Check sheet for the modelled part. Datum: model origin and axes. Units: mm. Face numbers are marked on the shaded views. A direction names the side the tool comes from. Give positions to 0.01 mm unless a question says otherwise; leave off trailing zeros. Order: outer loops, then holes, each group sorted by start corner. A loop starts at its lowest first (then second) coordinate and runs counter-clockwise, first axis right, second up.
Item 1: Gauge pin test, flat ends, axial feed: P1, Ø2, axis at y = 22.5, z = -3, coming from the +X side; P2, Ø3, axis at x = -14, z = -1, coming from the -Y side; P3, Ø1, axis at x = -16.5, y = 25.5, coming from the +Z side; P4, Ø3, axis at x = -1.5, z = -2.5, coming from the +Y side. Record the tip position at first contact, or that the pin passes through.
Item 2: Sectioned sample at A-A on y = 0. Record the boundary of the cut face in (x, z), and give its area (3 significant figures).
Item 3: Sectioned sample at B-B on x = 0. Record the boundary of the cut face in (y, z), and give its area (3 significant figures).
Item 4: Sectioned sample at C-C on z = -2. Record the boundary of the cut face in (x, y).
Item 5: Material ranges on line 1 along X through (y, z) = (0, -0.9); line 2 along Y through (x, z) = (0, -5.2); line 3 along Y through (x, z) = (0, -1.7), recorded low to high.
Item 6: Sectioned sample at D-D on x = -12.5. Record the boundary of the cut face in (y, z).
Item 7: Access from +Z, -Z, +X, -X, +Y, -Y to the whole of each face (thin tool, end or side, straight path). Record for the marked faces 1, 2 and 3.
Item 8: Release check for a two-part mould opening along Y. For the marked faces 4, 5, 6 and 7 record: released by +Y, released by -Y, zero draft, split by the parting line, or undercut.
from build123d import *

# Parameters (mm, degrees)
BOSS_EXTRUDE1_DEPTH = 6
FILLET1_R           = 5
FILLET2_R           = 15
FILLET3_R           = 5
FILLET4_R           = 5
FILLET5_R           = 3
FILLET6_R           = 3
CUT_EXTRUDE1_DEPTH  = 4.5
SKETCH3_R           = 1.5
CUT_EXTRUDE2_DEPTH  = 5


with BuildPart() as part:
    # Sketch2 → Boss-Extrude1 (new body)
    with BuildSketch(Plane.XY):
        Polygon((-14, 6), (6, 6), (6, -6), (-24, -6), (-24, 6), (-24, 36), (-14, 36), align=None)
    extrude(amount=-BOSS_EXTRUDE1_DEPTH)

    # Fillet1
    fillet1_edges = [part.edges().sort_by_distance(p)[0] for p in [
        (-14, 6, -3),
    ]]
    fillet(fillet1_edges, radius=FILLET1_R)

    # Fillet2
    fillet2_edges = [part.edges().sort_by_distance(p)[0] for p in [
        (-24, -6, -3),
    ]]
    fillet(fillet2_edges, radius=FILLET2_R)

    # Fillet3
    fillet3_edges = [part.edges().sort_by_distance(p)[0] for p in [
        (6, 6, -3),
    ]]
    fillet(fillet3_edges, radius=FILLET3_R)

    # Fillet4
    fillet4_edges = [part.edges().sort_by_distance(p)[0] for p in [
        (6, -6, -3),
    ]]
    fillet(fillet4_edges, radius=FILLET4_R)

    # Fillet5
    fillet5_edges = [part.edges().sort_by_distance(p)[0] for p in [
        (-14, 36, -3),
    ]]
    fillet(fillet5_edges, radius=FILLET5_R)

    # Fillet6
    fillet6_edges = [part.edges().sort_by_distance(p)[0] for p in [
        (-24, 36, -3),
    ]]
    fillet(fillet6_edges, radius=FILLET6_R)

    # Sketch1 → Cut-Extrude1 (cut)
    with BuildSketch(Plane.XY):
        with BuildLine():
            Line((-14.343060397, 1.923598719), (-2.139626136, 2.92))
            ThreePointArc((-2.139626136, 2.92), (3.62, 0), (-2.139626136, -2.92))
            Line((-2.139626136, -2.92), (-14.343060397, -1.923598719))
            ThreePointArc((-14.343060397, -1.923598719), (-16.116, 0), (-14.343060397, 1.923598719))
        make_face()
    extrude(amount=-CUT_EXTRUDE1_DEPTH, mode=Mode.SUBTRACT)

    # Sketch3 → Cut-Extrude2 (cut)
    with BuildSketch(Plane.XY.offset(-4.5)):
        Circle(SKETCH3_R)
    extrude(amount=-CUT_EXTRUDE2_DEPTH, mode=Mode.SUBTRACT)


solid = part.part
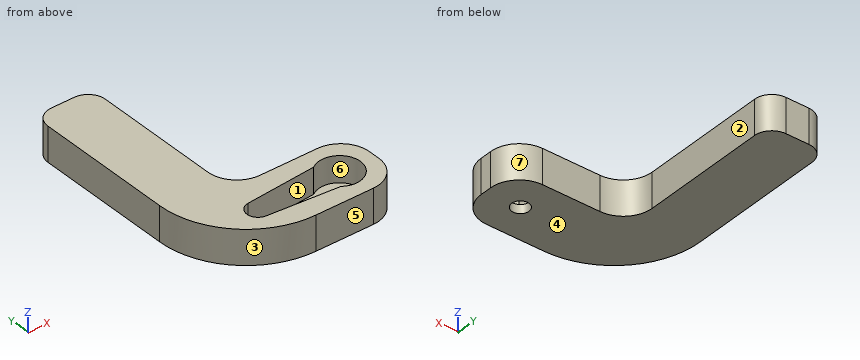
Report:
1. P1: stops at x = -14
1. P2: stops at y = -5.59
1. P3: stops at z = 0
1. P4: stops at y = 6
2. outline: (-21, -6) - (-1.5, -6) - (-1.5, -4.5) - (-16.12, -4.5) - (-16.12, 0) - (-21, 0) - close; (1.5, -6) - (6, -6) - (6, 0) - (3.62, 0) - (3.62, -4.5) - (1.5, -4.5) - close
2. area: 68.7 mm2
3. outline: (-6, -6) - (-1.5, -6) - (-1.5, -4.5) - (-3.62, -4.5) - (-3.62, 0) - (-6, 0) - close; (1.5, -6) - (6, -6) - (6, 0) - (3.62, 0) - (3.62, -4.5) - (1.5, -4.5) - close
3. area: 34.9 mm2
4. outline: (-24, 9) arc R15 ccw to (-9, -6) - (1, -6) arc R5 ccw to (6, -1) - (6, 1) arc R5 ccw to (1, 6) - (-9, 6) arc R5 cw to (-14, 11) - (-14, 33) arc R3 ccw to (-17, 36) - (-21, 36) arc R3 ccw to (-24, 33) - close; hole (-14.34, -1.92) - (-2.14, -2.92) arc R3.62 ccw (long way) to (-2.14, 2.92) - (-14.34, 1.92) arc R1.93 ccw to start
5. line 1: x = -21 to -16.12, 3.62 to 6
5. line 2: y = -6 to -1.5, 1.5 to 6
5. line 3: y = -6 to -3.62, 3.62 to 6
6. outline: (-5.59, -6) - (7.43, -6) - (7.43, 0) - (2.07, 0) - (2.07, -4.5) - (-2.07, -4.5) - (-2.07, 0) - (-5.59, 0) - close
7. face 1: +Z
7. face 2: +Z, -Z, +X, +Y
7. face 3: +Z, -Z, -X, -Y
8. face 4: zero draft
8. face 5: released by -Y
8. face 6: undercut
8. face 7: released by +Y
